For this review, take the finished solid that the model builds, in its own axes (mm). A direction names the side the tool comes from. Round coordinates to 2 decimals unless told otherwise and drop trailing zeros. Write each loop counter-clockwise with the first axis right and the second up, starting at its lowest first coordinate (ties: lowest second). Pieces come first, ordered by that corner, then holes. Notation, with made-up numbers: (8, 40.5) - (21, 40.5) arc R14 ccw to (21, 64.5) - close; hole circle Ø9 at (-6.75, 60). An arc over 180 degrees is marked (long way). One line per item, written item: value. Start each with the question number.
Q1. For probe 1 along X at (y, z) = (21, 0.1); probe 2 along Y at (x, z) = (31, 0.7); probe 3 along Y at (x, z) = (46, 1.05), list the stretches that pass through material, from the lowest coordinate up.
Q2. Add section C-C on z = 1.15. Give the number of separate pieces and of enclosed holes in the cut face, and give its area (3 significant figures).
Q3. Add section D-D on y = -9. Write out the cut boundary in (x, z), and give its area (3 significant figures).
Q4. Tool access review of faces 4 (the face through (38, 0, 2)), 5 (the face through (30, -16.9, 1)): name each direction out of +Z, -Z, +X, -X, +Y, -Y from which nothing blocks a thin tool from reaching the whole face with its end or side.
Q5. Clearance check with flat-ended pins moving along their axes: pin 1 Ø4 at (x, y) = (34.77, -5) entering from -Z; pin 2 Ø1.5 at (x, y) = (38, -1.5) entering from -Z. State where each tip first meets the part, or that it passes through.
Q6. Add section B-B on y = 4.5. Write out the cut boundary in (x, z).
Q7. Add section A-A on y = -21.5. Write out the cut boundary in (x, z).
Q8. Mouldability with a two-part tool opening along X and no side actions: class faces 1 (the face through (42.616, 0, 1)), 2 (the face through (44, 2.05, 1)), 3 (the face through (43.716, 20, 1)) as +X half, -X half, draft (parallel to the pull), parting line (faces both ways), or undercut.
```python
from build123d import *

# Parameters (mm, degrees)
SKETCH_1_R      = 2.55
SKETCH_1_R_2    = 2.05
SKETCH_1_W      = 6.2
SKETCH_1_H      = 6.2
EXTRUDE_1_DEPTH = 2


with BuildPart() as part:
    # 草图1 → 凸台-拉伸1 (new body)
    with BuildSketch(Plane.XY):
        with BuildLine():
            Line((53.016222961, -26), (23.516222961, -26))
            Line((23.516222961, -26), (23.516222961, -16.9))
            ThreePointArc((23.516222961, -16.9), (28.210668367, 0), (23.516222961, 16.9))
            Line((23.516222961, 16.9), (23.516222961, 26))
            Line((23.516222961, 26), (53.016222961, 26))
            Line((53.016222961, 26), (53.016222961, 2.05))
            Line((53.016222961, 2.05), (49.016222961, 2.05))
            Line((49.016222961, 2.05), (49.016222961, 3.5))
            Line((49.016222961, 3.5), (45.816222961, 3.5))
            Line((45.816222961, 3.5), (45.816222961, 2.05))
            Line((45.816222961, 2.05), (42.616222961, 2.05))
            Line((42.616222961, 2.05), (42.616222961, -2.05))
            Line((42.616222961, -2.05), (45.816222961, -2.05))
            Line((45.816222961, -2.05), (45.816222961, -3.5))
            Line((45.816222961, -3.5), (49.016222961, -3.5))
            Line((49.016222961, -3.5), (49.016222961, -2.05))
            Line((49.016222961, -2.05), (53.016222961, -2.05))
            Line((53.016222961, -2.05), (53.016222961, -26))
        make_face()
        with Locations((34.766222961, 5)):
            Circle(SKETCH_1_R, mode=Mode.SUBTRACT)
        with Locations((38.129788434, -18)):
            Circle(SKETCH_1_R_2, mode=Mode.SUBTRACT)
        with Locations(Location((34.766222961, -5, 0), (0, 0, 180))):
            Circle(SKETCH_1_R, mode=Mode.SUBTRACT)
        with Locations(Location((38.129788434, 18, 0), (0, 0, 180))):
            Circle(SKETCH_1_R_2, mode=Mode.SUBTRACT)
        with Locations((46.816222961, -20)):
            Rectangle(SKETCH_1_W, SKETCH_1_H, mode=Mode.SUBTRACT)
        with Locations((29.716222961, -20)):
            Rectangle(SKETCH_1_W, SKETCH_1_H, mode=Mode.SUBTRACT)
        with Locations((29.716222961, 20)):
            Rectangle(SKETCH_1_W, SKETCH_1_H, mode=Mode.SUBTRACT)
        with Locations((46.816222961, 20)):
            Rectangle(SKETCH_1_W, SKETCH_1_H, mode=Mode.SUBTRACT)
    extrude(amount=EXTRUDE_1_DEPTH)


solid = part.part
```
Result set:
1. probe 1: x = 23.52 to 26.62, 32.82 to 43.72, 49.92 to 53.02
1. probe 2: y = -26 to -23.1, -16.9 to 16.9, 23.1 to 26
1. probe 3: y = -26 to -23.1, -16.9 to -3.5, 3.5 to 16.9, 23.1 to 26
2. separate pieces: 1
2. enclosed holes: 8
2. area: 1,150 mm^2
3. outline: (26.95, 0) - (53.02, 0) - (53.02, 2) - (26.95, 2) - close
3. area: 52.1 mm^2
4. face 4: +Z, +X, -X, +Y, -Y
4. face 5: +Z, -Z
5. pin 1: passes through
5. pin 2: stops at z = 0
6. outline: (27.9, 0) - (32.27, 0) - (32.27, 2) - (27.9, 2) - close; (37.27, 0) - (53.02, 0) - (53.02, 2) - (37.27, 2) - close
7. outline: (23.52, 0) - (26.62, 0) - (26.62, 2) - (23.52, 2) - close; (32.82, 0) - (43.72, 0) - (43.72, 2) - (32.82, 2) - close; (49.92, 0) - (53.02, 0) - (53.02, 2) - (49.92, 2) - close
8. face 1: +X half
8. face 2: draft
8. face 3: undercut
